```python
from build123d import *

# Parameters (mm, degrees)
SKETCH1_R            = 12.5
BOSS_EXTRUDE1_DEPTH  = 4.4
SKETCH2_R            = 12.15
BOSS_EXTRUDE2_DEPTH  = 0.1
BOSS_EXTRUDE3_START  = 16
SKETCH3_R            = 12.5
BOSS_EXTRUDE3_DEPTH  = 16
SKETCH4_R            = 12.15
BOSS_EXTRUDE4_DEPTH  = 0.1
BOSS_EXTRUDE5_START  = 4.4
SKETCH5_R            = 12.5
BOSS_EXTRUDE5_DEPTH  = 4.4
SKETCH6_R            = 12.15
BOSS_EXTRUDE6_DEPTH  = 0.1
BOSS_EXTRUDE7_START  = 28.2
SKETCH7_R            = 12.5
BOSS_EXTRUDE7_DEPTH  = 28.2
SKETCH8_R            = 12.15
BOSS_EXTRUDE8_DEPTH  = 0.1
BOSS_EXTRUDE9_START  = 2.4
SKETCH9_R            = 12.5
BOSS_EXTRUDE9_DEPTH  = 2.4
SKETCH10_R           = 11.5
CUT_EXTRUDE1_DEPTH   = 0.8
SKETCH11_W           = 0.5
SKETCH11_H           = 3
BOSS_EXTRUDE10_DEPTH = 5
SKETCH12_R           = 0.75
CUT_EXTRUDE2_DEPTH   = 61.733927915
FILLET1_R            = 1
SKETCH13_R           = 1.25
CUT_EXTRUDE3_DEPTH   = 8
SKETCH14_R           = 3.5
BOSS_EXTRUDE11_DEPTH = 2.38
SKETCH15_R           = 2
BOSS_EXTRUDE12_DEPTH = 10
CUT_EXTRUDE4_START   = -8
CUT_EXTRUDE4_DEPTH   = 8
FILLET2_R            = 0.5


with BuildPart() as part:
    # Sketch1 → Boss-Extrude1 (new body)
    with BuildSketch(Plane(origin=(0, 0, 0), x_dir=(1, 0, 0), z_dir=(0, 1, 0))):
        with Locations(Location((0, 0, 0), (0, 0, 270))):
            Circle(SKETCH1_R)
    extrude(amount=BOSS_EXTRUDE1_DEPTH)

    # Sketch2 → Boss-Extrude2 (add)
    with BuildSketch(Plane.XZ):
        with Locations(Location((0, 0, 0), (0, 0, 270))):
            Circle(SKETCH2_R)
    extrude(amount=BOSS_EXTRUDE2_DEPTH)

    # Sketch3 → Boss-Extrude3 (add)
    with BuildSketch(Plane.XZ.offset(0.1).offset(BOSS_EXTRUDE3_START)):
        with Locations(Location((0, 0, 0), (0, 0, 90))):
            Circle(SKETCH3_R)
    extrude(amount=-BOSS_EXTRUDE3_DEPTH)

    # Sketch4 → Boss-Extrude4 (add)
    with BuildSketch(Plane.XZ.offset(16.1)):
        with Locations(Location((0, 0, 0), (0, 0, 270))):
            Circle(SKETCH4_R)
    extrude(amount=BOSS_EXTRUDE4_DEPTH)

    # Sketch5 → Boss-Extrude5 (add)
    with BuildSketch(Plane.XZ.offset(16.2).offset(BOSS_EXTRUDE5_START)):
        with Locations(Location((0, 0, 0), (0, 0, 90))):
            Circle(SKETCH5_R)
    extrude(amount=-BOSS_EXTRUDE5_DEPTH)

    # Sketch6 → Boss-Extrude6 (add)
    with BuildSketch(Plane.XZ.offset(20.6)):
        with Locations(Location((0, 0, 0), (0, 0, 270))):
            Circle(SKETCH6_R)
    extrude(amount=BOSS_EXTRUDE6_DEPTH)

    # Sketch7 → Boss-Extrude7 (add)
    with BuildSketch(Plane.XZ.offset(20.7).offset(BOSS_EXTRUDE7_START)):
        with Locations(Location((0, 0, 0), (0, 0, 90))):
            Circle(SKETCH7_R)
    extrude(amount=-BOSS_EXTRUDE7_DEPTH)

    # Sketch8 → Boss-Extrude8 (add)
    with BuildSketch(Plane.XZ.offset(48.9)):
        with Locations(Location((0, 0, 0), (0, 0, 270))):
            Circle(SKETCH8_R)
    extrude(amount=BOSS_EXTRUDE8_DEPTH)

    # Sketch9 → Boss-Extrude9 (add)
    with BuildSketch(Plane.XZ.offset(49).offset(BOSS_EXTRUDE9_START)):
        with Locations(Location((0, 0, 0), (0, 0, 90))):
            Circle(SKETCH9_R)
    extrude(amount=-BOSS_EXTRUDE9_DEPTH)

    # Sketch10 → Cut-Extrude1 (cut)
    with BuildSketch(Plane.XZ.offset(51.4)):
        with Locations(Location((0, 0, 0), (0, 0, 270))):
            Circle(SKETCH10_R)
    extrude(amount=-CUT_EXTRUDE1_DEPTH, mode=Mode.SUBTRACT)

    # Sketch11 → Boss-Extrude10 (add)
    with BuildSketch(Plane.XZ.offset(50.6)):
        with Locations((-8.25, 0)):
            Rectangle(SKETCH11_W, SKETCH11_H)
        with Locations((8.25, 0)):
            Rectangle(SKETCH11_W, SKETCH11_H)
    extrude(amount=BOSS_EXTRUDE10_DEPTH)

    # Sketch12 → Cut-Extrude2 (cut, through all)
    with BuildSketch(Plane(origin=(8.5, 0, 0), x_dir=(0, 0, -1), z_dir=(1, 0, 0))):
        with Locations((0, -54.4)):
            Circle(SKETCH12_R)
    extrude(amount=-CUT_EXTRUDE2_DEPTH, mode=Mode.SUBTRACT)

    # Fillet1
    fillet1_edges = [part.edges().sort_by_distance(p)[0] for p in [
        (-8.25, -55.6, 1.5),
        (-8.25, -55.6, -1.5),
        (8.25, -55.6, -1.5),
        (8.25, -55.6, 1.5),
    ]]
    fillet(fillet1_edges, radius=FILLET1_R)

    # Sketch13 → Cut-Extrude3 (cut)
    with BuildSketch(Plane(origin=(0, 4.4, 0), x_dir=(1, 0, 0), z_dir=(0, 1, 0))):
        with Locations(Location((0, 8.5, 0), (0, 0, 270))):
            Circle(SKETCH13_R)
        with Locations(Location((0, -8.5, 0), (0, 0, 90))):
            Circle(SKETCH13_R)
    extrude(amount=-CUT_EXTRUDE3_DEPTH, mode=Mode.SUBTRACT)

    # Sketch14 → Boss-Extrude11 (add)
    with BuildSketch(Plane(origin=(0, 4.4, 0), x_dir=(1, 0, 0), z_dir=(0, 1, 0))):
        with Locations(Location((0, 0, 0), (0, 0, 270))):
            Circle(SKETCH14_R)
    extrude(amount=BOSS_EXTRUDE11_DEPTH)

    # Sketch15 → Boss-Extrude12 (add)
    with BuildSketch(Plane(origin=(0, 6.78, 0), x_dir=(1, 0, 0), z_dir=(0, 1, 0))):
        with Locations(Location((0, 0, 0), (0, 0, 270))):
            Circle(SKETCH15_R)
    extrude(amount=BOSS_EXTRUDE12_DEPTH)

    # Sketch16 → Cut-Extrude4 (cut)
    with BuildSketch(Plane(origin=(0, 16.78, 0), x_dir=(1, 0, 0), z_dir=(0, 1, 0)).offset(CUT_EXTRUDE4_START)):
        with BuildLine():
            Line((-1.322875656, 1.5), (1.322875656, 1.5))
            ThreePointArc((1.322875656, 1.5), (0, 2), (-1.322875656, 1.5))
        make_face()
    extrude(amount=CUT_EXTRUDE4_DEPTH, mode=Mode.SUBTRACT)

    # Fillet2
    fillet2_edges = [part.edges().sort_by_distance(p)[0] for p in [
        (0, 4.4, -3.5),
        (0, 6.78, -3.5),
        (0, 4.4, -12.5),
    ]]
    fillet(fillet2_edges, radius=FILLET2_R)


solid = part.part
```
Can you work these out from the model? Positions are in its coordinate system, mm. A direction names the side the tool comes from. Coordinates: 2 decimals unless noted, no trailing zeros. Order: outer loops, then holes, each group sorted by start corner. A loop starts at its lowest first (then second) coordinate and runs counter-clockwise, first axis right, second up.
1. I need wall thicknesses on line 1 (X direction, y = -51.2, z = 0); line 2 (Y direction, x = -8.35, z = 0); line 3 (Z direction, x = 8.3, y = -54.4). Which ranges of each line are inside material? Lowest first, please.
2. If we section it at C-C (y = -42.5): Please give me the cut outline in (x, z).
3. If we section it at A-A (y = 1.5): Please give me the cut outline in (x, z).
4. Thinking about a two-plate mould opening in Y: for faces 4 (the face through (11, -51.4, 4)), 5 (the face through (-8.247, -55.065, -0.346)), 6 (the face through (-3.755, -18.431, 11.923)), 7 (the face through (0, -3.6, -9)), which applies, +Y half, -Y half, draft (parallel to the pull), parting line (faces both ways), or undercut?
5. For faces 1 (the face through (3.755, 1.923, 11.923)), 2 (the face through (3, 4.4, -3)), 3 (the face through (8, -53, 0)), which set-ups out of +Z, -Z, +X, -X, +Y, -Y let a thin tool reach every point of the face, with its end or its side?
6. If we section it at B-B (y = 9.5): Please give me the cut outline in (x, z).
7. I'm going to push flat-ended pins straight in: pin 1 (2 mm diameter, centred on y = -45.5, z = -4.5, fed in from -X); pin 2 (1.5 mm diameter, centred on x = 0, z = -8.5, fed in from +Y); pin 3 (5 mm diameter, centred on x = 0.5, z = 8, fed in from +Y). Where does each tip first touch, or does it pass through?
Entries:
1. line 1: x = -12.5 to -11.5, -8.5 to -8, 8 to 8.5, 11.5 to 12.5
1. line 2: y = -55.6 to -55.15, -53.65 to 4.4
1. line 3: z = -1.5 to -0.75, 0.75 to 1.5
2. outline: circle Ø25 at (0, 0)
3. outline: circle Ø25 at (0, 0); hole circle Ø2.5 at (0, -8.5); hole circle Ø2.5 at (0, 8.5)
4. face 4: -Y half
4. face 5: undercut
4. face 6: draft
4. face 7: +Y half
5. face 1: +Y, -Y
5. face 2: +Y
5. face 3: -Y
6. outline: (-1.32, -1.5) - (1.32, -1.5) arc R2 ccw (long way) to start
7. pin 1: stops at x = -12
7. pin 2: stops at y = -3.6
7. pin 3: stops at y = 4.4
